The model under review builds one solid part; all positions refer to its coordinate system, in mm. A direction names the side the tool comes from. Coordinates: 2 decimals unless noted, no trailing zeros. Write each loop counter-clockwise with the first axis right and the second up, starting at its lowest first coordinate (ties: lowest second). Pieces come first, ordered by that corner, then holes. Notation, with made-up numbers: (74, 68.25) -> (84, 68.25) arc R25 cw to (84, 89.25) -> close; hole circle Ø6 at (41.25, 37). An arc over 180 degrees is marked (long way). Write each question's results on one line, items separated by ' | '.
```python
from build123d import *

# Parameters (mm, degrees)
SKETCH1_W                        = 25.4
SKETCH1_H                        = 5.08
BOSS_EXTRUDE1_DEPTH              = 2.54
BOSS_EXTRUDE5_DEPTH              = 2.54
SKETCH6_R                        = 1.27
BOSS_EXTRUDE6_DEPTH              = 1
BOSS_EXTRUDE7_DEPTH              = 1
SKETCH8_W                        = 25.4
SKETCH8_H                        = 8
BOSS_EXTRUDE8_DEPTH              = 2.54
SKETCH11_R                       = 0.5
CUT_EXTRUDE1_DEPTH               = 17.24
CUT_EXTRUDE2_DEPTH               = 10.54
SKETCH2_W                        = 1
SKETCH2_H                        = 4.46
BOSS_EXTRUDE2_DEPTH              = 2.54
SKETCH13_R                       = 0.75
BOSS_EXTRUDE12_DEPTH             = 3.08
CUT_EXTRUDE3_DEPTH               = 9
BOSS_EXTRUDE13_REACH             = 12.16
SKETCH16_R                       = 0.45
BOSS_EXTRUDE13_DIRECTION_2_REACH = 17.24


with BuildPart() as part:
    # Sketch1 → Boss-Extrude1 (new body)
    with BuildSketch(Plane(origin=(0, 0, 0), x_dir=(1, 0, 0), z_dir=(0, 1, 0))):
        Rectangle(SKETCH1_W, SKETCH1_H)
    extrude(amount=BOSS_EXTRUDE1_DEPTH)

    # Sketch5 → Boss-Extrude5 (add)
    with BuildSketch(Plane(origin=(0, 2.54, 0), x_dir=(1, 0, 0), z_dir=(0, 1, 0))):
        Polygon((-3.54, 2.54), (-3.54, -2.54), (-2.54, -2.54), (-2.54, -7.62), (-1.54, -7.62), (-1.54, -1.482742514), (-2.54, -1.482742514), (-2.54, 2.54), align=None)
    boss_extrude5 = extrude(amount=BOSS_EXTRUDE5_DEPTH)

    # Sketch6 → Boss-Extrude6 (add)
    with BuildSketch(Plane(origin=(-1.54, 0, 0), x_dir=(0, 0, -1), z_dir=(1, 0, 0))):
        with Locations((-7.62, 3.81)):
            Circle(SKETCH6_R)
    boss_extrude6 = extrude(amount=-BOSS_EXTRUDE6_DEPTH)

    # Sketch7 → Boss-Extrude7 (add)
    with BuildSketch(Plane(origin=(-2.54, 0, 0), x_dir=(0, 0, -1), z_dir=(1, 0, 0))):
        with BuildLine():
            Line((2.54, 5.08), (2.54, 2.54))
            ThreePointArc((2.54, 2.54), (3.81, 3.81), (2.54, 5.08))
        make_face()
    boss_extrude7 = extrude(amount=-BOSS_EXTRUDE7_DEPTH)

    # Mirror1: Boss-Extrude5, Boss-Extrude6, Boss-Extrude7 across plane
    add(boss_extrude5.mirror(Plane(origin=(0, 0, 0), x_dir=(0, 0, 1), z_dir=(1, 0, 0))))
    add(boss_extrude6.mirror(Plane(origin=(0, 0, 0), x_dir=(0, 0, 1), z_dir=(1, 0, 0))))
    add(boss_extrude7.mirror(Plane(origin=(0, 0, 0), x_dir=(0, 0, 1), z_dir=(1, 0, 0))))

    # Sketch8 → Boss-Extrude8 (add)
    with BuildSketch(Plane.XZ.offset(-2.54)):
        with Locations((0, 1.46)):
            Rectangle(SKETCH8_W, SKETCH8_H)
    extrude(amount=BOSS_EXTRUDE8_DEPTH)

    # Sketch11 → Cut-Extrude1 (cut, through all)
    with BuildSketch(Plane(origin=(3.54, 0, 0), x_dir=(0, 0, -1), z_dir=(1, 0, 0))):
        with Locations((2.54, 3.81)):
            Circle(SKETCH11_R)
    extrude(amount=-CUT_EXTRUDE1_DEPTH, mode=Mode.SUBTRACT)

    # Sketch12 → Cut-Extrude2 (cut)
    with BuildSketch(Plane(origin=(3.54, 0, 0), x_dir=(0, 0, -1), z_dir=(1, 0, 0))):
        with BuildLine():
            Line((1.923817285, 5.08), (1.72030075, 5.08))
            Line((1.72030075, 5.08), (2.177926741, 4.101139391))
            ThreePointArc((2.177926741, 4.101139391), (2.54, 3.34539351), (2.902073259, 4.101139391))
            Line((2.902073259, 4.101139391), (3.256261376, 4.8587467))
            ThreePointArc((3.256261376, 4.8587467), (2.914827754, 5.023426617), (2.54, 5.08))
            Line((2.54, 5.08), (1.923817285, 5.08))
        make_face()
    extrude(amount=-CUT_EXTRUDE2_DEPTH, mode=Mode.SUBTRACT)

    # Sketch2 → Boss-Extrude2 (add)
    with BuildSketch(Plane(origin=(0, 2.54, 0), x_dir=(1, 0, 0), z_dir=(0, 1, 0))):
        with Locations((-3.04, -0.31)):
            Rectangle(SKETCH2_W, SKETCH2_H)
        with Locations((3.04, -0.31)):
            Rectangle(SKETCH2_W, SKETCH2_H)
    extrude(amount=BOSS_EXTRUDE2_DEPTH)

    # Sketch13 → Boss-Extrude12 (add)
    with BuildSketch(Plane.ZY.offset(-1.54)):
        with Locations((7.46, 3.81)):
            Circle(SKETCH13_R)
    extrude(amount=BOSS_EXTRUDE12_DEPTH)

    # Sketch14 → Cut-Extrude3 (cut)
    with BuildSketch(Plane(origin=(3.54, 0, 0), x_dir=(0, 0, -1), z_dir=(1, 0, 0))):
        Polygon((1.92, 4.652843909), (1.72030075, 5.08), (1.92, 5.08), align=None)
    extrude(amount=-CUT_EXTRUDE3_DEPTH, mode=Mode.SUBTRACT)

    # Boss-Extrude13: up to this face of the body (flat: up to its plane)
    boss_extrude13_end = Plane(part.part.faces().sort_by_distance((-3.54, 3.747341049, -0.245716728))[0])
    # Sketch16 → Boss-Extrude13 (add, up to the picked face)
    with BuildSketch(Plane.ZY.offset(2.54), mode=Mode.PRIVATE) as boss_extrude13_sk1:
        with Locations((7.46, 3.81)):
            Circle(SKETCH16_R)
    boss_extrude13_tool1 = split(extrude(boss_extrude13_sk1.sketch, amount=BOSS_EXTRUDE13_REACH, mode=Mode.PRIVATE), bisect_by=boss_extrude13_end, keep=Keep.BOTH, mode=Mode.PRIVATE)
    add(boss_extrude13_tool1.solids().sort_by_distance((-2.54, 3.81, 7.46))[0])

    # Boss-Extrude13 direction 2: up to this face of the body (flat: up to its plane)
    boss_extrude13_direction_2_end = Plane(part.part.faces().sort_by_distance((3.54, 3.747341049, -0.245716728))[0])
    # Sketch16 → Boss-Extrude13 direction 2 (add, up to the picked face)
    with BuildSketch(Plane.ZY.offset(2.54), mode=Mode.PRIVATE) as boss_extrude13_direction_2_sk1:
        with Locations((7.46, 3.81)):
            Circle(SKETCH16_R)
    boss_extrude13_direction_2_tool1 = split(extrude(boss_extrude13_direction_2_sk1.sketch, amount=-BOSS_EXTRUDE13_DIRECTION_2_REACH, mode=Mode.PRIVATE), bisect_by=boss_extrude13_direction_2_end, keep=Keep.BOTH, mode=Mode.PRIVATE)
    add(boss_extrude13_direction_2_tool1.solids().sort_by_distance((-2.54, 3.81, 7.46))[0])


solid = part.part
```
Q1. Clearance check with flat-ended pins moving along their axes: P1, Ø0.8, axis at x = 2, z = 7, coming from the -Y side; P2, Ø2.5, axis at x = -8, z = 0.5, coming from the +Y side; P3, Ø1.5, axis at x = 8, z = 7, coming from the -Y side; P4, Ø1.5, axis at y = 3.5, z = 5.5, coming from the +X side. State where each tip first meets the part, or that it passes through.
Solution:
P1: y = 2.54 | P2: y = 2.54 | P3: through | P4: x = 2.54
Q2. Add section A-A (x = -3). Write out the cut boundary in (y, z).
Solution:
outline: (0, -2.54) -> (2.54, -2.54) arc R1.27 ccw to (4.86, -3.26) -> (4.14, -2.92) arc R0.5 cw (long way) to (4.14, -2.16) -> (5.08, -1.72) -> (5.08, 2.54) -> (2.54, 2.54) -> (2.54, 5.46) -> (0, 5.46) -> close; circle Ø0.9 at (3.81, 7.46)
Q3. For line 1 (Z direction, x = -2.85, y = 3.81); line 2 (X direction, y = 4.4, z = 4.5); line 3 (X direction, y = 3.65, z = -2), list the stretches that pass through material, from the lowest coordinate up. Write a range as from..to.
Solution:
line 1: -3.81..-3.04, -2.04..2.54, 7.01..7.91 | line 2: -2.54..-1.54, 1.54..2.54 | line 3: -3.54..-2.54, 2.54..3.54
Q4. Add section C-C (z = 2.25). Write out the cut boundary in (x, y), plus the area to 3 significant figures.
Solution:
outline: (-12.7, 0) -> (12.7, 0) -> (12.7, 2.54) -> (3.54, 2.54) -> (3.54, 5.08) -> (1.54, 5.08) -> (1.54, 2.54) -> (-1.54, 2.54) -> (-1.54, 5.08) -> (-3.54, 5.08) -> (-3.54, 2.54) -> (-12.7, 2.54) -> close | area: 74.7 mm²
Q5. Machinability: for faces 1 (the flat face through (-2.54, 4, -1)), 2 (the flat face through (2, 2.54, 7)), 3 (the flat face through (0, 1, -2.54)), which of the approach directions +Z, -Z, +X, -X, +Y, -Y give a long, thin tool a straight path to every point of the face, cutting with its end or side? Answer none if there is none.
Solution:
face 1: -Z, +Y | face 2: +Z, +X, -X, -Y | face 3: -Z, +X, -X, -Y
Q6. Add section D-D (y = 3.81). Count the separate pieces of the cut face and the enclosed holes in it, plus the area to 3 significant figures.
Solution:
separate pieces: 3 | enclosed holes: 0 | area: 31.9 mm²
Q7. Draft analysis for pull direction Z (two halves, no side actions). For faces 4 (the flat face through (-3.54, 4, -1)), 5 (the cylindrical face through (3.05, 3.31, -2.52)), 6 (the cylindrical face through (0.02, 3.52, 8.15)), state which applies: pulls with the +Z half, pulls with the -Z half, needs draft (parallel to the pull), parting line crosses it, or undercut.
Solution:
face 4: needs draft | face 5: undercut | face 6: parting line crosses it
Q8. Add section B-B (z = 6). Write out the cut boundary in (x, y).
Solution:
outline: (-2.54, 2.54) -> (-1.54, 2.54) -> (-1.54, 5.08) -> (-2.54, 5.08) -> close; (1.54, 2.54) -> (2.54, 2.54) -> (2.54, 5.08) -> (1.54, 5.08) -> close
